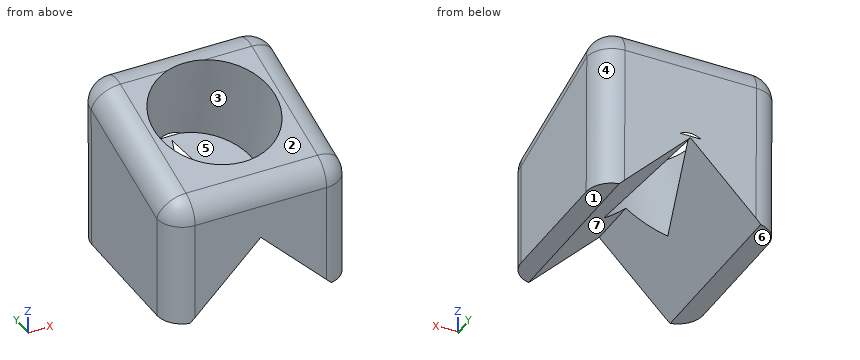
```python
from build123d import *

# Parameters (mm, degrees)
F1_DEPTH     = 18
F2_R         = 12
F3_DEPTH     = 20
F5_DEPTH     = 19
F6_T1_DEPTH  = 33.0501766006
F6_T3_DEPTH  = 26
F6_T5_DEPTH  = 26.4486901769
F6_T7_DEPTH  = 40.9649172436
F6_T12_DEPTH = 5
F6_T18_DEPTH = 5
F6_T24_DEPTH = 5
F6_T30_DEPTH = 5


# Not quite as in the source:
# - a fillet or chamfer that OpenCascade refuses, or shapes differently, is made with other operations: its cross-section is extruded or revolved along the edge and cut away or added


with BuildPart() as f1:
    # F0 (on Right) → F1 (new body, symmetric)
    with BuildSketch(Plane.YZ):
        Polygon((-17.5945106894, -16.5027584881), (17.4054893106, -16.5027584881), (17.6841049034, 18.8368745636), (-17.5945106894, 7.7135697939), align=None)
    extrude(amount=F1_DEPTH, both=True)

    # F2 (on face) → F3 (cut)
    with BuildSketch(Plane(origin=(0, -3.8031265819, 12.0619764999), x_dir=(1, 0, 0), z_dir=(0, -0.3007057995, 0.9537169507))):
        with Locations((0, 4.2350762524)):
            Circle(F2_R)
    extrude(amount=-F3_DEPTH, mode=Mode.SUBTRACT)

    # F4 (on Front) → F5 (cut, symmetric)
    with BuildSketch(Plane.XZ):
        Polygon((18.3847763109, -20.8875347989), (0, -2.5027584881), (-18.3847763109, -20.8875347989), (0, -39.2723111098), align=None)
    extrude(amount=F5_DEPTH, both=True, mode=Mode.SUBTRACT)

    # F6: fillet of radius 5 on 8 edges, made by hand

    # F6_s2 → F6_t1 (cut)
    with BuildSketch(Plane.XY.offset(-29.0027584881)):
        with BuildLine():
            ThreePointArc((-18, -12.5945106894), (-16.5355339059, -16.1300445953), (-13, -17.5945106894))
            Line((-13, -17.5945106894), (-18, -17.5945106894))
            Line((-18, -17.5945106894), (-18, -12.5945106894))
        make_face()
        with BuildLine():
            ThreePointArc((13, -17.5945106894), (16.5355339059, -16.1300445953), (18, -12.5945106894))
            Line((18, -12.5945106894), (18, -17.5945106894))
            Line((18, -17.5945106894), (13, -17.5945106894))
        make_face()
    extrude(amount=F6_T1_DEPTH, mode=Mode.SUBTRACT)

    # F6_s4 → F6_t3 (cut)
    with BuildSketch(Plane.YZ.offset(-13)):
        with BuildLine():
            ThreePointArc((-14.0980396869, 8.8160028663), (-16.6267337107, 7.0039663544), (-17.5945106894, 4.0474181125))
            Line((-17.5945106894, 4.0474181125), (-17.5945106894, 7.7135697939))
            Line((-17.5945106894, 7.7135697939), (-14.0980396869, 8.8160028663))
        make_face()
        with BuildLine():
            ThreePointArc((11.1265244599, 16.7692773918), (15.6024732635, 16.0212299773), (17.6298980733, 11.9612741565))
            Line((17.6298980733, 11.9612741565), (17.6841049034, 18.8368745636))
            Line((17.6841049034, 18.8368745636), (11.1265244599, 16.7692773918))
        make_face()
    extrude(amount=F6_T3_DEPTH, mode=Mode.SUBTRACT)

    # F6_s6 → F6_t5 (cut)
    with BuildSketch(Plane(origin=(0, 14.9296510418, 4.7073008919), x_dir=(1, 0, 0), z_dir=(0, -0.9537169507, -0.3007057995))):
        with BuildLine():
            ThreePointArc((-13, 12.6473336669), (-16.5355339059, 11.1828675728), (-18, 7.6473336669))
            Line((-18, 7.6473336669), (-18, 12.6473336669))
            Line((-18, 12.6473336669), (-13, 12.6473336669))
        make_face()
        with BuildLine():
            ThreePointArc((13, 12.6473336669), (16.5355339059, 11.1828675728), (18, 7.6473336669))
            Line((18, 7.6473336669), (18, 12.6473336669))
            Line((18, 12.6473336669), (13, 12.6473336669))
        make_face()
    extrude(amount=F6_T5_DEPTH, mode=Mode.SUBTRACT)

    # F6_s8 → F6_t7 (cut)
    with BuildSketch(Plane(origin=(0, -0.227563099, -28.8641290101), x_dir=(1, 0, 0), z_dir=(0, 0.0078836963, 0.9999689232))):
        with BuildLine():
            ThreePointArc((13, 17.5350511394), (16.5355339059, 16.0705850454), (18, 12.5350511394))
            Line((18, 12.5350511394), (18, 17.5350511394))
            Line((18, 17.5350511394), (13, 17.5350511394))
        make_face()
        with BuildLine():
            ThreePointArc((-18, 12.5350511394), (-16.5355339059, 16.0705850454), (-13, 17.5350511394))
            Line((-13, 17.5350511394), (-18, 17.5350511394))
            Line((-18, 17.5350511394), (-18, 12.5350511394))
        make_face()
    extrude(amount=F6_T7_DEPTH, mode=Mode.SUBTRACT)


with BuildPart() as f6_tool10:
    # F6_s11 → F6_t12 (new body)
    with BuildSketch(Plane.YZ.offset(-13)):
        Polygon((-12.5945106894, 4.0474181125), (-17.5945106894, 4.0474181125), (-17.5945106894, 7.7135697939), (-14.0980396869, 8.8160028663), align=None)
    extrude(amount=-F6_T12_DEPTH)

    # F6_s13 → F6_t14 (revolve, cut)
    with BuildSketch(Plane(origin=(-13, -12.5945106894, 4.0474181125), x_dir=(0, 0.8064446043, -0.5913096484), z_dir=(0, 0.5913096484, 0.8064446043))):
        with BuildLine():
            ThreePointArc((0, -5), (5, 0), (0, 5))
            Line((0, 5), (0, -5))
        make_face()
    revolve(axis=Axis((-13, -12.5945106894, 4.0474181125), (-1, 0, 0)), mode=Mode.SUBTRACT)


with BuildPart() as f1_1:
    add(f1.part)

    # F6_t9: cut F6_tool10
    add(f6_tool10.part, mode=Mode.SUBTRACT)


with BuildPart() as f6_tool16:
    # F6_s17 → F6_t18 (new body)
    with BuildSketch(Plane.YZ.offset(13)):
        Polygon((-12.5945106894, 4.0474181125), (-14.0980396869, 8.8160028663), (-17.5945106894, 7.7135697939), (-17.5945106894, 4.0474181125), align=None)
    extrude(amount=F6_T18_DEPTH)

    # F6_s19 → F6_t20 (revolve, cut)
    with BuildSketch(Plane(origin=(13, -12.5945106894, 4.0474181125), x_dir=(0, 0.8064446043, -0.5913096484), z_dir=(0, -0.5913096484, -0.8064446043))):
        with BuildLine():
            ThreePointArc((0, -5), (5, 0), (0, 5))
            Line((0, 5), (0, -5))
        make_face()
    revolve(axis=Axis((13, -12.5945106894, 4.0474181125), (1, 0, 0)), mode=Mode.SUBTRACT)


with BuildPart() as f1_2:
    add(f1_1.part)

    # F6_t15: cut F6_tool16
    add(f6_tool16.part, mode=Mode.SUBTRACT)


with BuildPart() as f6_tool22:
    # F6_s23 → F6_t24 (new body)
    with BuildSketch(Plane.YZ.offset(-13)):
        Polygon((12.6300534574, 12.000692638), (17.6298980733, 11.9612741565), (17.6841049034, 18.8368745636), (11.1265244599, 16.7692773918), align=None)
    extrude(amount=-F6_T24_DEPTH)

    # F6_s25 → F6_t26 (revolve, cut)
    with BuildSketch(Plane(origin=(-13, 12.6300534574, 12.000692638), x_dir=(0, -0.5944839612, -0.8041074679), z_dir=(0, 0.8041074679, -0.5944839612))):
        with BuildLine():
            ThreePointArc((0, -5), (5, 0), (0, 5))
            Line((0, 5), (0, -5))
        make_face()
    revolve(axis=Axis((-13, 12.6300534574, 12.000692638), (-1, 0, 0)), mode=Mode.SUBTRACT)


with BuildPart() as f1_3:
    add(f1_2.part)

    # F6_t21: cut F6_tool22
    add(f6_tool22.part, mode=Mode.SUBTRACT)


with BuildPart() as f6_tool28:
    # F6_s29 → F6_t30 (new body)
    with BuildSketch(Plane.YZ.offset(13)):
        Polygon((12.6300534574, 12.000692638), (11.1265244599, 16.7692773918), (17.6841049034, 18.8368745636), (17.6298980733, 11.9612741565), align=None)
    extrude(amount=F6_T30_DEPTH)

    # F6_s31 → F6_t32 (revolve, cut)
    with BuildSketch(Plane(origin=(13, 12.6300534574, 12.000692638), x_dir=(0, -0.5944839612, -0.8041074679), z_dir=(0, -0.8041074679, 0.5944839612))):
        with BuildLine():
            ThreePointArc((0, -5), (5, 0), (0, 5))
            Line((0, 5), (0, -5))
        make_face()
    revolve(axis=Axis((13, 12.6300534574, 12.000692638), (1, 0, 0)), mode=Mode.SUBTRACT)


with BuildPart() as f1_4:
    add(f1_3.part)

    # F6_t27: cut F6_tool28
    add(f6_tool28.part, mode=Mode.SUBTRACT)


solid = f1_4.part
```
Work out the finished part from the listing and answer in its coordinate system (mm). Face numbers are marked on the shaded views. A direction names the side the tool comes from. Round coordinates to 2 decimals unless told otherwise and drop trailing zeros. Write each loop counter-clockwise with the first axis right and the second up, starting at its lowest first coordinate (ties: lowest second). Pieces come first, ordered by that corner, then holes. Notation, with made-up numbers: (49.5, 17.25) - (95.5, 17.25) arc R24 ccw to (95.5, 31.25) - close; hole circle Ø9 at (59.25, 17.25). An arc over 180 degrees is marked (long way). Return JSON: item names as keys, results as strings. Group by question number.
Q1. The part is cut by section B-B on x = 9.5. Write down the section's boundary in (y, z), then the cut area to 3 significant figures.
Q2. The mould has two halves that part along Y. Classify the marked faces 1, 2 and 3: released by +Y, released by -Y, zero draft, split by the parting line, or undercut.
Q3. Find the intervals of material crossed by L1, parallel to X at y = 11, z = 4; L2, parallel to X at y = 12, z = -11.5; L3, parallel to Y at x = -9, z = 1.5, in increasing order.
Q4. For the marked faces 4, 5, 6 and 7, determine the directions among +Z, -Z, +X, -X, +Y, -Y from which every point of the face is accessible in a straight line to the end or side of a thin tool.
Q5. The part is cut by section A-A on x = 4.5. Write down the section's boundary in (y, z).
Q6. Each of these flat-tipped pins is pushed along its axis until it touches: pin 1 Ø12 at (x, y) = (-9.5, -13.5) entering from +Z; pin 2 Ø5 at (x, z) = (-12.5, -11) entering from +Y; pin 3 Ø8 at (x, y) = (8, -6) entering from +Z; pin 4 Ø6 at (x, z) = (-2.5, -12.5) entering from -Y. Where does it stop, or does it pass through?
Q7. The part is cut by section C-C on x = -10.5. Write down the section's boundary in (y, z).
Solved:
{
 "1": {"outline": "(-17.59, -12) - (17.44, -12) - (17.63, 11.96) arc R5 ccw to (11.13, 16.77) - (7.23, 15.54) - (13.24, -3.53) - (-0.74, -7.94) - (-6.76, 11.13) - (-14.1, 8.82) arc R5 ccw to (-17.59, 4.05) - close", "area": "581 mm²"},
 "2": {"face 1": "zero draft", "face 2": "released by -Y", "face 3": "undercut"},
 "3": {"L1": "-18 to -9.4, 9.4 to 18", "L2": "-18 to -9, 9 to 18", "L3": "-17.59 to -4.35, 12.29 to 17.55"},
 "4": {"face 4": "-Z, +X, +Y", "face 5": "none", "face 6": "-Z, +X, -X, +Y, -Y", "face 7": "-Z, +Y, -Y"},
 "5": {"outline": "(-17.59, -7) - (-5.02, -7) - (-10.37, 9.99) - (-14.1, 8.82) arc R5 ccw to (-17.59, 4.05) - close; (2.24, -7) - (17.48, -7) - (17.63, 11.96) arc R5 ccw to (11.13, 16.77) - (10.85, 16.68) - (16.86, -2.39) - close"},
 "6": {"pin 1": "z = 10.9", "pin 2": "y = 17.47", "pin 3": "z = 12.1", "pin 4": "through"},
 "7": {"outline": "(-17.59, -13) - (17.43, -13) - (17.63, 11.96) arc R5 ccw to (11.13, 16.77) - (5.78, 15.08) - (11.79, -3.99) - (0.71, -7.49) - (-5.3, 11.59) - (-14.1, 8.82) arc R5 ccw to (-17.59, 4.05) - close"}
}
